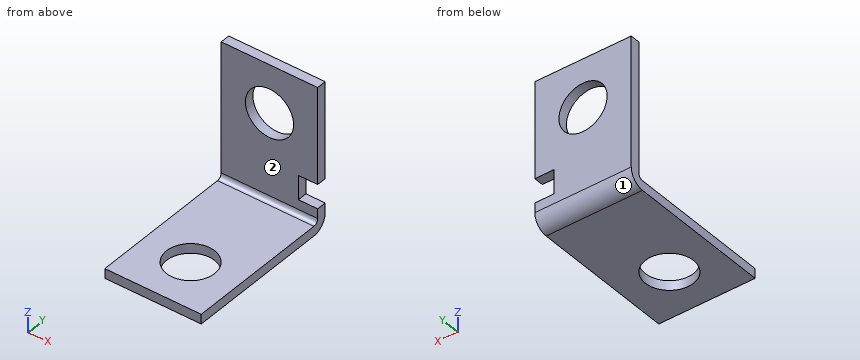
from build123d import *

# Parameters (mm, degrees)
F1_DEPTH = 20
F2_R     = 5
F2_W     = 4
F2_H     = 5
F3_DEPTH = 25
F4_R     = 5
F5_DEPTH = 25


with BuildPart() as f1:
    # F0 (on Right) → F1 (new body)
    with BuildSketch(Plane.YZ):
        with BuildLine():
            Line((0, 2), (0, 0))
            Line((0, 0), (30, 0))
            ThreePointArc((30, 0), (32.12132, 0.87868), (33, 3))
            Line((33, 3), (33, 30))
            Line((33, 30), (31, 30))
            Line((31, 30), (31, 3))
            ThreePointArc((31, 3), (30.707107, 2.292893), (30, 2))
            Line((30, 2), (0, 2))
        make_face()
    extrude(amount=F1_DEPTH)

    # F2 (on face) → F3 (cut)
    with BuildSketch(Plane.XZ.offset(-31)):
        with Locations((10, 20)):
            Circle(F2_R)
        with Locations((18, 7.5)):
            Rectangle(F2_W, F2_H)
    extrude(amount=-F3_DEPTH, mode=Mode.SUBTRACT)

    # F4 (on face) → F5 (cut)
    with BuildSketch(Plane.XY.offset(2)):
        with Locations((10, 10)):
            Circle(F4_R)
    extrude(amount=-F5_DEPTH, mode=Mode.SUBTRACT)


solid = f1.part
Model file for the job. Use its own axes, mm. Face numbers are marked on the shaded views. A direction names the side the tool comes from. Give positions to 0.01 mm unless a question says otherwise; leave off trailing zeros. Order: outer loops, then holes, each group sorted by start corner. A loop starts at its lowest first (then second) coordinate and runs counter-clockwise, first axis right, second up. Notation, with made-up numbers: (77.5, 25) - (99.5, 25) arc R4 ccw to (99.5, 31) - close; hole circle Ø6 at (65.5, -15.75). An arc over 180 degrees is marked (long way). One line per item, written item: value.
Item 1: Tool access for the marked faces 1 and 2: list every direction of +Z, -Z, +X, -X, +Y, -Y with a clear straight run to the whole face (end or side of a thin tool).
Response values:
face 1: -Z, +X, -X, +Y
face 2: +Z, +X, -X, -Y
Item 2: Pin check, flat tips, straight feed: pin 1 Ø8 at (x, z) = (9.5, 24) entering from -Y; pin 2 Ø1.5 at (x, y) = (17.5, 22.5) entering from +Z; pin 3 Ø1 at (x, y) = (19, 32.5) entering from -Z; pin 4 Ø12 at (y, z) = (20.5, 16) entering from +X. Stop position of each tip, or through.
Response values:
pin 1: y = 31
pin 2: z = 2
pin 3: z = 0.76
pin 4: through
Item 3: Slice it at D-D (x = 3.5). List the corners of the cut face in (y, z).
Response values:
outline: (0, 0) - (30, 0) arc R3 ccw to (33, 3) - (33, 30) - (31, 30) - (31, 3) arc R1 cw to (30, 2) - (0, 2) - close
Item 4: Wall check: line 1 (Y direction, x = 9.5, z = 4); line 2 (Z direction, x = 12.75, y = 22); line 3 (Z direction, x = 10, y = 32.4). Give the ranges that are in metal, low to high.
Response values:
line 1: 31 to 33
line 2: 0 to 2
line 3: 1.2 to 15, 25 to 30
Item 5: Slice it at B-B (x = 10). List the corners of the cut face in (y, z), then the cut area to 3 significant figures.
Response values:
outline: (0, 0) - (5, 0) - (5, 2) - (0, 2) - close; (15, 0) - (30, 0) arc R3 ccw to (33, 3) - (33, 15) - (31, 15) - (31, 3) arc R1 cw to (30, 2) - (15, 2) - close; (31, 25) - (33, 25) - (33, 30) - (31, 30) - close
area: 80.3 mm2
Item 6: Slice it at C-C (y = 10). List the corners of the cut face in (x, z).
Response values:
outline: (0, 0) - (5, 0) - (5, 2) - (0, 2) - close; (15, 0) - (20, 0) - (20, 2) - (15, 2) - close
Item 7: Slice it at A-A (z = 20). List the corners of the cut face in (x, y), then the cut area to 3 significant figures.
Response values:
outline: (0, 31) - (5, 31) - (5, 33) - (0, 33) - close; (15, 31) - (20, 31) - (20, 33) - (15, 33) - close
area: 20.0 mm2
